Design review of the part built by this model. Coordinates are the model's own, in mm. Coordinates: 2 decimals unless noted, no trailing zeros. Loops run counter-clockwise (first coordinate to the right, second up) from the corner with the lowest first, then second, coordinate; pieces in that order, holes last. Notation, with made-up numbers: (6, 66.25) -> (58, 66.25) arc R15 ccw to (58, 78.25) -> close; hole circle Ø2 at (-33.5, 61.5). An arc over 180 degrees is marked (long way). Use a Markdown table: item, result. Add a question column.
Q1. Take a section at A-A on z = 0. Write out the cut boundary in (x, y), plus the area to 4 significant figures.
Q2. For probe 1 along Z at (x, y) = (0, -0.5); probe 2 along X at (y, z) = (2.5, 0); probe 3 along X at (y, z) = (0.75, 0), list the stretches that pass through material, from the lowest coordinate up.
Q3. Take a section at B-B on x = 0. Write out the cut boundary in (y, z), plus the area to 4 significant figures.
Q4. Clearance check with flat-ended pins moving along their axes: pin 1 Ø2.5 at (x, z) = (-22.74, -62.49) entering from -Y; pin 2 Ø4 at (x, y) = (7.5, -0.5) entering from +Z; pin 3 Ø4 at (x, y) = (-55.5, 0.5) entering from +Z; pin 4 Ø4 at (x, y) = (4.5, -3.5) entering from -Z. State where each tip first meets the part, or that it passes through.
Q5. Take a section at D-D on x = -33.25. Write out the cut boundary in (y, z).
Q6. Take a section at C-C on x = -51. Write out the cut boundary in (y, z).
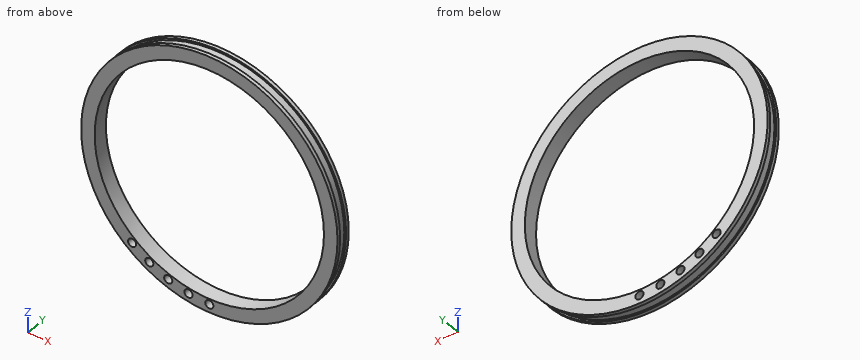
from build123d import *

# Parameters (mm, degrees)
SKETCH1_R               = 70
BOSS_EXTRUDE1_DEPTH     = 2.25
SKETCH2_R               = 71
BOSS_EXTRUDE2_DEPTH     = 2
SKETCH3_R               = 63.5
CUT_EXTRUDE1_DEPTH      = 1
CUT_EXTRUDE1_DEPTH_BACK = 9.5
SKETCH5_R               = 2.25
CUT_EXTRUDE3_DEPTH      = 5.25
CIRPATTERN1_COUNT       = 5
CIRPATTERN1_ANGLE       = 40


with BuildPart() as part:
    # Sketch1 → Boss-Extrude1 (new body, symmetric)
    with BuildSketch(Plane(origin=(0, 0, 0), x_dir=(1, 0, 0), z_dir=(0, 1, 0))):
        Circle(SKETCH1_R)
    extrude(amount=BOSS_EXTRUDE1_DEPTH, both=True)

    # Sketch2 → Boss-Extrude2 (add)
    with BuildSketch(Plane(origin=(0, 2.25, 0), x_dir=(1, 0, 0), z_dir=(0, 1, 0))):
        Circle(SKETCH2_R)
    boss_extrude2 = extrude(amount=BOSS_EXTRUDE2_DEPTH)

    # Mirror1: Boss-Extrude2 across plane
    add(boss_extrude2.mirror(Plane.ZX))

    # Sketch3 → Cut-Extrude1 (cut, two sides)
    with BuildSketch(Plane(origin=(0, 4.25, 0), x_dir=(1, 0, 0), z_dir=(0, 1, 0))) as cut_extrude1_sk:
        Circle(SKETCH3_R)
    extrude(amount=CUT_EXTRUDE1_DEPTH, mode=Mode.SUBTRACT)
    extrude(cut_extrude1_sk.sketch, amount=-CUT_EXTRUDE1_DEPTH_BACK, mode=Mode.SUBTRACT)

    # Sketch5 → Cut-Extrude3 (cut, symmetric)
    with BuildSketch(Plane(origin=(0, 0, 0), x_dir=(1, 0, 0), z_dir=(0, 1, 0))):
        with Locations((0, 66.5)):
            Circle(SKETCH5_R)
    cut_extrude3 = extrude(amount=CUT_EXTRUDE3_DEPTH, both=True, mode=Mode.SUBTRACT)

    # CirPattern1: Cut-Extrude3 ×5 about axis
    cirpattern1_axis = Axis((0, 0, 0), (0, 1, 0))
    for i in range(1, CIRPATTERN1_COUNT):
        add(cut_extrude3.rotate(cirpattern1_axis, i * CIRPATTERN1_ANGLE / (CIRPATTERN1_COUNT - 1)), mode=Mode.SUBTRACT)


solid = part.part
Answer list:
| question | item | result |
|---|---|---|
| 1 | outline | (-71, -4.25) -> (-63.5, -4.25) -> (-63.5, 4.25) -> (-71, 4.25) -> (-71, 2.25) -> (-70, 2.25) -> (-70, -2.25) -> (-71, -2.25) -> close; (63.5, -4.25) -> (71, -4.25) -> (71, -2.25) -> (70, -2.25) -> (70, 2.25) -> (71, 2.25) -> (71, 4.25) -> (63.5, 4.25) -> close |
| 1 | area | 118.5 mm² |
| 2 | probe 1 | -70 to -68.75, -64.25 to -63.5, 63.5 to 70 |
| 2 | probe 2 | -71 to -63.5, 63.5 to 71 |
| 2 | probe 3 | -70 to -63.5, 63.5 to 70 |
| 3 | outline | (-4.25, -71) -> (-2.25, -71) -> (-2.25, -70) -> (2.25, -70) -> (2.25, -71) -> (4.25, -71) -> (4.25, -68.75) -> (-4.25, -68.75) -> close; (-4.25, -64.25) -> (4.25, -64.25) -> (4.25, -63.5) -> (-4.25, -63.5) -> close; (-4.25, 63.5) -> (4.25, 63.5) -> (4.25, 71) -> (2.25, 71) -> (2.25, 70) -> (-2.25, 70) -> (-2.25, 71) -> (-4.25, 71) -> close |
| 3 | area | 80.25 mm² |
| 4 | pin 1 | through |
| 4 | pin 2 | z = 70.7 |
| 4 | pin 3 | z = 45.47 |
| 4 | pin 4 | z = -70.96 |
| 5 | outline | (-4.25, -62.73) -> (-2.25, -62.73) -> (-2.25, -61.6) -> (2.25, -61.6) -> (2.25, -62.73) -> (4.25, -62.73) -> (4.25, -59.84) -> (-4.25, -59.84) -> close; (-4.25, -55.34) -> (4.25, -55.34) -> (4.25, -54.1) -> (-4.25, -54.1) -> close; (-4.25, 54.1) -> (4.25, 54.1) -> (4.25, 62.73) -> (2.25, 62.73) -> (2.25, 61.6) -> (-2.25, 61.6) -> (-2.25, 62.73) -> (-4.25, 62.73) -> close |
| 6 | outline | (-4.25, -49.4) -> (-2.25, -49.4) -> (-2.25, -47.95) -> (2.25, -47.95) -> (2.25, -49.4) -> (4.25, -49.4) -> (4.25, -37.83) -> (-4.25, -37.83) -> close; (-4.25, 37.83) -> (4.25, 37.83) -> (4.25, 49.4) -> (2.25, 49.4) -> (2.25, 47.95) -> (-2.25, 47.95) -> (-2.25, 49.4) -> (-4.25, 49.4) -> close |
